from build123d import *

# Parameters (mm, degrees)
SKETCH_1_R          = 28.7
SKETCH_1_R_2        = 1.5
EXTRUDE_1_DEPTH     = 3
EXTRUDE_START       = -48
SKETCH_2_R          = 34.7
SKETCH_2_R_2        = 28.7
EXTRUDE_2_DEPTH     = 48
SKETCH_3_W          = 12
SKETCH_3_H          = 23
CUT_EXTRUDE_1_DEPTH = 10
FILLET_1_R          = 2
SKETCH_4_W          = 30
SKETCH_4_H          = 25
CUT_EXTRUDE_2_DEPTH = 96.094431221
FILLET_2_R          = 2
SKETCH_5_W          = 160
SKETCH_5_H          = 90
SKETCH_5_R          = 34.7
SKETCH_5_R_2        = 1.5
EXTRUDE_3_DEPTH     = 5.5
SKETCH_7_R          = 2.05
CUT_EXTRUDE_3_DEPTH = 104.580886314
FILLET_4_R          = 8
CUT_EXTRUDE_START   = -3
SKETCH_8_R          = 3.5
SKETCH_8_R_2        = 1.5
CUT_EXTRUDE_4_DEPTH = 3
SKETCH_9_R          = 34.7
CUT_EXTRUDE_5_DEPTH = 48


with BuildPart() as part:
    # 草图1 → 凸台-拉伸1 (new body)
    with BuildSketch(Plane.XY):
        Circle(SKETCH_1_R)
        with Locations((0, 19)):
            Circle(SKETCH_1_R_2, mode=Mode.SUBTRACT)
        with Locations((19, 0)):
            Circle(SKETCH_1_R_2, mode=Mode.SUBTRACT)
        with Locations((0, -19)):
            Circle(SKETCH_1_R_2, mode=Mode.SUBTRACT)
        with Locations((-19, 0)):
            Circle(SKETCH_1_R_2, mode=Mode.SUBTRACT)
    extrude(amount=EXTRUDE_1_DEPTH)

    # 草图2 → 凸台-拉伸2 (add)
    with BuildSketch(Plane.XY.offset(3).offset(EXTRUDE_START)):
        Circle(SKETCH_2_R)
        Circle(SKETCH_2_R_2, mode=Mode.SUBTRACT)
    extrude(amount=EXTRUDE_2_DEPTH)

    # 草图3 → 切除-拉伸1 (cut)
    with BuildSketch(Plane(origin=(-24.536605307, 24.536605307, 0), x_dir=(0, 0, 1), z_dir=(-0.7071067811865488, 0.7071067811865464, 0))):
        with Locations((-6, 0)):
            Rectangle(SKETCH_3_W, SKETCH_3_H)
    extrude(amount=-CUT_EXTRUDE_1_DEPTH, mode=Mode.SUBTRACT)

    # 圆角1
    fillet_1_edges = [part.edges().sort_by_distance(p)[0] for p in [
        (-12.740018652, 29.00347462, -12),
        (-12.740018652, 29.00347462, 0),
        (-29.00347462, 12.740018652, 0),
        (-29.00347462, 12.740018652, -12),
    ]]
    fillet(fillet_1_edges, radius=FILLET_1_R)

    # 草图4 → 切除-拉伸2 (cut, through all)
    with BuildSketch(Plane(origin=(24.536605307, 24.536605307, 0), x_dir=(0.7071067811865487, -0.7071067811865465, 0), z_dir=(0.7071067811865465, 0.7071067811865487, 0))):
        with Locations((0.808951296, 22.5)):
            Rectangle(SKETCH_4_W, SKETCH_4_H)
    extrude(amount=-CUT_EXTRUDE_2_DEPTH, mode=Mode.SUBTRACT)

    # 圆角2
    fillet_2_edges = [part.edges().sort_by_distance(p)[0] for p in [
        (-8.211322504, -30.568555834, -35),
        (30.568555834, 8.211322504, -35),
        (-8.211322504, -30.568555834, -10),
        (30.568555834, 8.211322504, -10),
        (-30.049784568, -9.980611027, -10),
        (9.980611027, 30.049784568, -10),
        (-30.049784568, -9.980611027, -35),
        (9.980611027, 30.049784568, -35),
    ]]
    fillet(fillet_2_edges, radius=FILLET_2_R)

    # 草图5 → 凸台-拉伸3 (add)
    # profile 1 of 2: a face of its own
    with BuildSketch(Plane.XY.offset(3)):
        Rectangle(SKETCH_5_W, SKETCH_5_H)
        Circle(SKETCH_5_R, mode=Mode.SUBTRACT)
    # profile 2 of 2: a face of its own
    with BuildSketch(Plane.XY.offset(3)):
        Circle(SKETCH_5_R)
        with Locations((0, 19)):
            Circle(SKETCH_5_R_2, mode=Mode.SUBTRACT)
        with Locations((-19, 0)):
            Circle(SKETCH_5_R_2, mode=Mode.SUBTRACT)
        with Locations((19, 0)):
            Circle(SKETCH_5_R_2, mode=Mode.SUBTRACT)
        with Locations((0, -19)):
            Circle(SKETCH_5_R_2, mode=Mode.SUBTRACT)
    extrude(amount=EXTRUDE_3_DEPTH)

    # 草图7 → 切除-拉伸3 (cut, through all)
    with BuildSketch(Plane(origin=(0, 0, 3), x_dir=(-1, 0, 0), z_dir=(0, 0, -1))):
        with Locations((-72, 37)):
            Circle(SKETCH_7_R)
        with Locations((72, 37)):
            Circle(SKETCH_7_R)
        with Locations((72, -37)):
            Circle(SKETCH_7_R)
        with Locations((-72, -37)):
            Circle(SKETCH_7_R)
    extrude(amount=-CUT_EXTRUDE_3_DEPTH, mode=Mode.SUBTRACT)

    # 圆角4
    fillet_4_edges = [part.edges().sort_by_distance(p)[0] for p in [
        (80, -45, 5.75),
        (80, 45, 5.75),
        (-80, 45, 5.75),
        (-80, -45, 5.75),
    ]]
    fillet(fillet_4_edges, radius=FILLET_4_R)

    # 草图8 → 切除-拉伸4 (cut)
    # profile 1 of 4: a face of its own
    with BuildSketch(Plane.XY.offset(8.5).offset(CUT_EXTRUDE_START)):
        with Locations((-19, 0)):
            Circle(SKETCH_8_R)
        with Locations((-19, 0)):
            Circle(SKETCH_8_R_2, mode=Mode.SUBTRACT)
    # profile 2 of 4: a face of its own
    with BuildSketch(Plane.XY.offset(8.5).offset(CUT_EXTRUDE_START)):
        with Locations((0, 19)):
            Circle(SKETCH_8_R)
    # profile 3 of 4: a face of its own
    with BuildSketch(Plane.XY.offset(8.5).offset(CUT_EXTRUDE_START)):
        with Locations((19, 0)):
            Circle(SKETCH_8_R)
    # profile 4 of 4: a face of its own
    with BuildSketch(Plane.XY.offset(8.5).offset(CUT_EXTRUDE_START)):
        with Locations((0, -19)):
            Circle(SKETCH_8_R)
    extrude(amount=CUT_EXTRUDE_4_DEPTH, mode=Mode.SUBTRACT)

    # 草图9 → 切除-拉伸5 (cut)
    with BuildSketch(Plane(origin=(0, 0, -45), x_dir=(-1, 0, 0), z_dir=(0, 0, -1))):
        Circle(SKETCH_9_R)
    extrude(amount=-CUT_EXTRUDE_5_DEPTH, mode=Mode.SUBTRACT)


solid = part.part
The model under review builds one solid part; all positions refer to its coordinate system, in mm. A direction names the side the tool comes from. Coordinates: 2 decimals unless noted, no trailing zeros. Write each loop counter-clockwise with the first axis right and the second up, starting at its lowest first coordinate (ties: lowest second). Pieces come first, ordered by that corner, then holes. Notation, with made-up numbers: M 58,-10 L 103,-10 A26 cw 103,19 Z; hole C 31.25,-13.75 d8. An arc over 180 degrees is marked long. Put each result on its own line as item: value.
1) Clearance check with a flat-ended pin moving along its axis: pin 1 Ø6.5 at (x, y) = (19, 0) entering from +Z. State where the tip first meets the part, or that it passes through.
Computed:
pin 1: stops at z = 5.5
2) Wall thickness on probe 1 along X at (y, z) = (0, 4.7); probe 2 along Y at (x, z) = (0, 4.4); probe 3 along Y at (x, z) = (-72, 5.25): over which ranges is each line inside the solid? List them lowest first. Write a range as [from, to].
Computed:
probe 1: x = [-80, -20.5], [-17.5, 17.5], [20.5, 80]
probe 2: y = [-45, -20.5], [-17.5, 17.5], [20.5, 45]
probe 3: y = [-45, -39.05], [-34.95, 34.95], [39.05, 45]
3) Add section A-A on y = -19. Give the boundary of the cut face in (x, z), then the cut area to 4 significant figures.
Computed:
outline: M -80,3 L -1.5,3 L -1.5,5.5 L -3.5,5.5 L -3.5,8.5 L -80,8.5 Z; M 1.5,3 L 80,3 L 80,8.5 L 3.5,8.5 L 3.5,5.5 L 1.5,5.5 Z
area: 851.5 mm2
4) Add section B-B on x = -19. Give the boundary of the cut face in (y, z), then the cut area to 4 significant figures.
Computed:
outline: M -45,3 L -1.5,3 L -1.5,5.5 L -3.5,5.5 L -3.5,8.5 L -45,8.5 Z; M 1.5,3 L 45,3 L 45,8.5 L 3.5,8.5 L 3.5,5.5 L 1.5,5.5 Z
area: 466.5 mm2
5) For faces 1 (the cylindrical face through (73.5, -35.6, 5.7)), 2 (the cylindrical face through (22.34, 1.05, 6.98)), list the 3-axis set-ups (+Z, -Z, +X, -X, +Y, -Y) from which the entire face can be reached by the end or side of a thin tool; tool diameter is ignored.
Computed:
face 1: +Z, -Z
face 2: +Z
6) Add section C-C on y = 0. Give the boundary of the cut face in (x, z), then the cut area to 3 significant figures.
Computed:
outline: M -80,3 L -20.5,3 L -20.5,5.5 L -22.5,5.5 L -22.5,8.5 L -80,8.5 Z; M -17.5,3 L 17.5,3 L 17.5,5.5 L 15.5,5.5 L 15.5,8.5 L -15.5,8.5 L -15.5,5.5 L -17.5,5.5 Z; M 20.5,3 L 80,3 L 80,8.5 L 22.5,8.5 L 22.5,5.5 L 20.5,5.5 Z
area: 823 mm2
7) Add section D-D on x = 0. Give the boundary of the cut face in (y, z).
Computed:
outline: M -45,3 L -20.5,3 L -20.5,5.5 L -22.5,5.5 L -22.5,8.5 L -45,8.5 Z; M -17.5,3 L 17.5,3 L 17.5,5.5 L 15.5,5.5 L 15.5,8.5 L -15.5,8.5 L -15.5,5.5 L -17.5,5.5 Z; M 20.5,3 L 45,3 L 45,8.5 L 22.5,8.5 L 22.5,5.5 L 20.5,5.5 Z
